Work out the finished part from the listing and answer in its coordinate system (mm). A direction names the side the tool comes from. Round coordinates to 2 decimals unless told otherwise and drop trailing zeros. Loops run counter-clockwise (first coordinate to the right, second up) from the corner with the lowest first, then second, coordinate; pieces in that order, holes last. Notation, with made-up numbers: (88, 27) -> (107, 27) arc R20 ccw to (107, 65) -> close; hole circle Ø5 at (42.25, 21). An arc over 180 degrees is marked (long way). Use CSV: the item, a comma, the result in double quotes. Start each with the question number.
Autodesk Inventor part; units mm, degrees
ref_plane "YZ Plane" through (0, 0, 0) normal (1, 0, 0) x (0, 1, 0)
ref_plane "XZ Plane" through (0, 0, 0) normal (0, 1, 0) x (-1, 0, 0)
ref_plane "XY Plane" through (0, 0, 0) normal (0, 0, 1) x (1, 0, 0)
sketch "Sketch1" plane through (0, 0, 0) normal (0, 0, 1) x (1, 0, 0)
  line L0 (-75, -40) -> (75, -40)
  line L1 (75, -40) -> (75, 40)
  line L2 (75, 40) -> (-75, 40)
  line L3 (-75, 40) -> (-75, -40)
  line L4 (-75, -40) -> (75, 40) construction
  line L5 (75, -40) -> (-75, 40) construction
  point P0 (0, 0)
  dimension "d0" = 150
  dimension "d1" = 80
extrude "Extrusion1" add sketch "Sketch1" along normal blind 5
sketch "Sketch4" plane through (0, 0, 5) normal (0, 0, 1) x (1, 0, 0)
  line L0 (-60, -20) -> (40, -20)
  line L1 (40, -20) -> (40, 20)
  line L2 (40, 20) -> (-60, 20)
  line L3 (-60, 20) -> (-60, -20)
  line L4 (-60, -20) -> (40, 20) construction
  line L5 (40, -20) -> (-60, 20) construction
  point P0 (0, 0)
  point P1 (-10, 0)
  point P2 (-10, 0)
  dimension "d8" = 100
  dimension "d9" = 40
  dimension "d10" = 10
extrude "Extrusion3" cut sketch "Sketch4" against normal through all
sketch "Sketch5" plane through (0, 0, 5) normal (0, 0, 1) x (1, 0, 0)
  line L0 (40, 20) -> (40, -20)
  point P0 (0, 0)
  point P1 (55, 0)
  dimension "d13" = 15
hole "Hole1" at (55, 0, 5) direction (0, 0, -1) diameter 9 depth 8 tip angle 118
sketch "Sketch6" plane through (0, 0, 5) normal (0, 0, 1) x (1, 0, 0)
  line L0 (-56.5, -27.5) -> (36.5, -27.5) construction
  line L1 (36.5, -27.5) -> (36.5, 27.5) construction
  line L2 (36.5, 27.5) -> (-56.5, 27.5) construction
  line L3 (-56.5, 27.5) -> (-56.5, -27.5) construction
  line L4 (-56.5, -27.5) -> (36.5, 27.5) construction
  line L5 (36.5, -27.5) -> (-56.5, 27.5) construction
  point P0 (0, 0)
  point P1 (-10, 0)
  point P2 (-10, 0)
  dimension "d21" = 93
  dimension "d22" = 55
  dimension "d23" = 10
hole "Hole2" at (-56.5, 27.5, 5) at (36.5, 27.5, 5) at (36.5, -27.5, 5) at (-56.5, -27.5, 5) direction (0, 0, -1) diameter 3.4 depth 8 tip angle 118
fillet "Fillet1" radius 2 4 edges at (-60, 20, 2.5) (-60, -20, 2.5) (40, -20, 2.5) (40, 20, 2.5)
fillet "Fillet2" radius 4 4 edges at (75, 40, 2.5) (-75, 40, 2.5) (75, -40, 2.5) (-75, -40, 2.5)
sketch "Sketch7" plane through (0, 0, 5) normal (0, 0, 1) x (1, 0, 0)
  line L0 (-50, 33) -> (50, 33) construction
  line L1 (50, 33) -> (50, 38) construction
  line L2 (50, 38) -> (-50, 38) construction
  line L3 (-50, 38) -> (-50, 33) construction
  line L4 (50, -38) -> (-50, -38) construction
  line L5 (-50, -38) -> (-50, -33) construction
  line L6 (-50, -33) -> (50, -33) construction
  line L7 (50, -33) -> (50, -38) construction
  line L8 (71, 40) -> (-71, 40)
  line L9 (-71, -40) -> (71, -40)
  line L10 (-50, 33) -> (-10, 33)
  line L11 (-10, 33) -> (-10, 38)
  line L12 (-10, 38) -> (-50, 38)
  line L13 (-50, 38) -> (-50, 33)
  line L14 (50, 33) -> (10, 33)
  line L15 (10, 33) -> (10, 38)
  line L16 (10, 38) -> (50, 38)
  line L17 (50, 38) -> (50, 33)
  line L18 (50, -38) -> (10, -38)
  line L19 (10, -38) -> (10, -33)
  line L20 (10, -33) -> (50, -33)
  line L21 (50, -33) -> (50, -38)
  line L22 (-50, -38) -> (-10, -38)
  line L23 (-10, -38) -> (-10, -33)
  line L24 (-10, -33) -> (-50, -33)
  line L25 (-50, -33) -> (-50, -38)
  point P0 (0, 0)
  point P1 (0, 38)
  dimension "d33" = 5
  dimension "d34" = 5
  dimension "d35" = 100
  dimension "d36" = 2
  dimension "d37" = 2
  dimension "d38" = 20
  dimension "d39" = 20
  dimension "d40" = 10
  dimension "d41" = 10
extrude "Extrusion4" cut sketch "Sketch7" against normal blind 5
sketch "Sketch8" plane through (0, 0, 5) normal (0, 0, 1) x (1, 0, 0)
  line L0 (-50, -33) -> (-10, -33)
  line L1 (-10, 33) -> (-50, 33)
  point P0 (0, 0)
  point P1 (0, 35.5)
  point P2 (0, -35.5)
  dimension "d44" = 2.5
  dimension "d45" = 2.5
hole "Hole3" at (0, 35.5, 5) at (0, -35.5, 5) direction (0, 0, -1) diameter 3.4 depth 8 tip angle 118
sketch "Sketch11" plane through (0, 0, 5) normal (0, 0, 1) x (1, 0, 0)
  circle A0 centre (55, 0) radius 4.5
  point P0 (0, 0)
  point P1 (55, 16)
  dimension "d53" = 16
hole "Hole4" at (55, 16, 5) direction (0, 0, -1) diameter 6.2 depth 8 tip angle 118
properties part number "Interrupter_Top" material "Polycarbonate, Clear"
Q1. Straight lines are drawn through the part: line 1 (X direction, y = -35.5, z = 3.7); line 2 (X direction, y = 0, z = 2.95); line 3 (X direction, y = -27.5, z = 3.9). For each, find the intervals that lie inside material, in ascending order. Write a range as from..to.
Q2. Section B-B, the plane y = -12 is taken. Write down the section's boundary in (x, z), and give its area (3 significant figures).
Q3. Which of the six approach directions +Z, -Z, +X, -X, +Y, -Y give full straight-line access (tool end or side, diameter ignored) to faces 1 (the cylindrical face through (-73.859, -38.797, 2.535)), 2 (the flat face through (-30, -38, 3))?
Q4. Section C-C, the plane x = -44 is taken. Write down the section's boundary in (y, z).
Q5. For a pull along Y with two mould halves and no side action, classify faces 3 (the flat face through (10, -36, 3)), 4 (the flat face through (1, 40, 2)), 5 (the flat face through (-75, 1, 2)) as pulls with the +Y half, pulls with the -Y half, needs draft (parallel to the pull), parting line crosses it, or undercut.
Q6. Section A-A, the plane x = 36.5 is taken. Write down the section's boundary in (y, z).
Q7. Section D-D, the plane y = 0 is taken. Write down the section's boundary in (x, z).
Report:
1,line 1,"x = -75..-50, -10..-1.7, 1.7..10, 50..75"
1,line 2,"x = -75..-60, 40..50.5, 59.5..75"
1,line 3,"x = -75..-58.2, -54.8..34.8, 38.2..75"
2,outline,"(-75, 0) -> (-60, 0) -> (-60, 5) -> (-75, 5) -> close; (40, 0) -> (75, 0) -> (75, 5) -> (40, 5) -> close"
2,area,"250 mm²"
3,face 1,"+Z, -Z, -X, -Y"
3,face 2,"+Z, -Z"
4,outline,"(-40, 0) -> (-38, 0) -> (-38, 5) -> (-40, 5) -> close; (-33, 0) -> (-20, 0) -> (-20, 5) -> (-33, 5) -> close; (20, 0) -> (33, 0) -> (33, 5) -> (20, 5) -> close; (38, 0) -> (40, 0) -> (40, 5) -> (38, 5) -> close"
5,face 3,"undercut"
5,face 4,"pulls with the +Y half"
5,face 5,"needs draft"
6,outline,"(-40, 0) -> (-38, 0) -> (-38, 5) -> (-40, 5) -> close; (-33, 0) -> (-29.2, 0) -> (-29.2, 5) -> (-33, 5) -> close; (-25.8, 0) -> (-20, 0) -> (-20, 5) -> (-25.8, 5) -> close; (20, 0) -> (25.8, 0) -> (25.8, 5) -> (20, 5) -> close; (29.2, 0) -> (33, 0) -> (33, 5) -> (29.2, 5) -> close; (38, 0) -> (40, 0) -> (40, 5) -> (38, 5) -> close"
7,outline,"(-75, 0) -> (-60, 0) -> (-60, 5) -> (-75, 5) -> close; (40, 0) -> (50.5, 0) -> (50.5, 5) -> (40, 5) -> close; (59.5, 0) -> (75, 0) -> (75, 5) -> (59.5, 5) -> close"
